For this review, take the finished solid that the model builds, in its own axes (mm). A direction names the side the tool comes from. Give positions to 0.01 mm unless a question says otherwise; leave off trailing zeros. Loops run counter-clockwise (first coordinate to the right, second up) from the corner with the lowest first, then second, coordinate; pieces in that order, holes last. Notation, with made-up numbers: (76, 10.25) -> (133, 10.25) arc R29 ccw to (133, 32.25) -> close; hole circle Ø1 at (21, 87). An arc over 180 degrees is marked (long way). Answer as CSV lines item,"result". Start each with the question number.
Item 1: Add section A-A on z = -142. State the section outline as (x, y) points.
Item 2: Clearance check with flat-ended pins moving along their axes: P1, Ø11.5, axis at y = 10, z = -51, coming from the +X side; P2, Ø4, axis at x = 6.5, z = -28, coming from the +Y side; P3, Ø2, axis at x = 13.5, z = -78.5, coming from the +Y side. State where each tip first meets the part, or that it passes through.
Item 3: The part is to be moulded in two halves that separate along X. For faces 1 (the face through (14, 23, 5)), 2 (the face through (-7.1, 22.18, 7.14)), 3 (the face through (2, 18, -180.976)), say which applies: +X half, -X half, draft (parallel to the pull), parting line (faces both ways), or undercut.
Item 4: Add section B-B on y = 7.5. State the section outline as (x, z) points.
Item 5: Add section C-C on x = 3. State the section outline as (y, z) points.
Item 6: Machinability: for faces 4 (the face through (0, 41, -92)), 5 (the face through (17.03, 18.25, -7.75)), 6 (the face through (19.976, 18, -2)), 7 (the face through (7.701, 18.252, -177.946)), which of the approach directions +Z, -Z, +X, -X, +Y, -Y give a long, thin tool a straight path to every point of the face, cutting with its end or side? Answer none if there is none.
Item 7: For L1, parallel to X at y = 11, z = -124.5; L2, parallel to Y at x = 0.5, z = -120.5; L3, parallel to Z at x = -3.75, y = 22, list the stretches that pass through material, from the lowest coordinate up. Write a range as from..to.
```python
from build123d import *

# Parameters (mm, degrees)
SKETCH_1_W                = 270
SKETCH_1_H                = 370
SKETCH_1_W_2              = 250
SKETCH_1_H_2              = 350
EXTRUDE_2_DEPTH           = 45
SKETCH_4_W                = 250
SKETCH_4_H                = 350
SKETCH_4_W_2              = 222
SKETCH_4_H_2              = 322
EXTRUDE_3_DEPTH           = 5
SKETCH_9_W                = 246
SKETCH_9_H                = 346
SKETCH_9_W_2              = 226
SKETCH_9_H_2              = 326
CUT_EXTRUDE_3_DEPTH       = 2.5
SKETCH_12_R               = 1.6
CUT_EXTRUDE_5_DEPTH       = 109.5
FILLET_1_R                = 5
SKETCH_13_W               = 250
SKETCH_13_H               = 350
SKETCH_13_W_2             = 222
SKETCH_13_H_2             = 322
EXTRUDE_4_DEPTH           = 33.5
CUT_EXTRUDE_START         = -126.5
SKETCH_14_R               = 1.6
CUT_EXTRUDE_9_DEPTH       = 126.5
SKETCH_15_R               = 1.6
CUT_EXTRUDE_10_DEPTH      = 50
CUT_EXTRUDE_11_DEPTH      = 2.5
CUT_EXTRUDE_12_DEPTH      = 188.55314569
CUT_EXTRUDE_12_DEPTH_BACK = 188.55314569


with BuildPart() as part:
    # 草图1 → 凸台-拉伸2 (new body)
    with BuildSketch(Plane(origin=(0, 0, 0), x_dir=(1, 0, 0), z_dir=(0, 1, 0))):
        with Locations((125, 175)):
            Rectangle(SKETCH_1_W, SKETCH_1_H)
        with Locations((125, 175)):
            Rectangle(SKETCH_1_W_2, SKETCH_1_H_2, mode=Mode.SUBTRACT)
    extrude(amount=EXTRUDE_2_DEPTH)

    # 草图4 → 凸台-拉伸3 (add)
    with BuildSketch(Plane(origin=(0, 38.5, 0), x_dir=(1, 0, 0), z_dir=(0, 1, 0))):
        with Locations((125, 175)):
            Rectangle(SKETCH_4_W, SKETCH_4_H)
        with Locations((125, 175)):
            Rectangle(SKETCH_4_W_2, SKETCH_4_H_2, mode=Mode.SUBTRACT)
    extrude(amount=-EXTRUDE_3_DEPTH)

    # 草图9 → 切除-拉伸3 (cut)
    with BuildSketch(Plane(origin=(0, 38.5, 0), x_dir=(1, 0, 0), z_dir=(0, 1, 0))):
        with Locations((125, 175)):
            Rectangle(SKETCH_9_W, SKETCH_9_H)
        with Locations((125, 175)):
            Rectangle(SKETCH_9_W_2, SKETCH_9_H_2, mode=Mode.SUBTRACT)
    extrude(amount=-CUT_EXTRUDE_3_DEPTH, mode=Mode.SUBTRACT)

    # 草图12 → 切除-拉伸5 (cut)
    with BuildSketch(Plane(origin=(0, 45, 0), x_dir=(1, 0, 0), z_dir=(0, 1, 0))):
        with Locations(Location((-3.535533906, -3.535533906, 0), (0, 0, 270))):
            Circle(SKETCH_12_R)
        with BuildLine():
            ThreePointArc((-4.666904756, 354.666904756), (-4.666904756, 352.404163056), (-2.404163056, 352.404163056))
            Line((-2.404163056, 352.404163056), (-4.666904756, 354.666904756))
        make_face()
        with BuildLine():
            Line((-4.666904756, 354.666904756), (-2.404163056, 352.404163056))
            ThreePointArc((-2.404163056, 352.404163056), (-2.057326654, 352.923240414), (-1.935533906, 353.535533906))
            ThreePointArc((-1.935533906, 353.535533906), (-2.923240414, 355.013741158), (-4.666904756, 354.666904756))
        make_face()
        with Locations(Location((253.535533906, 353.535533906, 0), (0, 0, 270))):
            Circle(SKETCH_12_R)
        with Locations(Location((253.535533906, -3.535533906, 0), (0, 0, 270))):
            Circle(SKETCH_12_R)
    extrude(amount=-CUT_EXTRUDE_5_DEPTH, mode=Mode.SUBTRACT)

    # 圆角1
    fillet_1_edges = [part.edges().sort_by_distance(p)[0] for p in [
        (-10, 22.5, 10),
        (-10, 22.5, -360),
        (260, 22.5, -360),
        (260, 22.5, 10),
    ]]
    fillet(fillet_1_edges, radius=FILLET_1_R)

    # 草图13 → 凸台-拉伸4 (add)
    with BuildSketch(Plane.XZ.offset(-33.5)):
        with Locations((125, -175)):
            Rectangle(SKETCH_13_W, SKETCH_13_H)
        with Locations((125, -175)):
            Rectangle(SKETCH_13_W_2, SKETCH_13_H_2, mode=Mode.SUBTRACT)
    extrude(amount=EXTRUDE_4_DEPTH)

    # 草图14 → 切除-拉伸9 (cut)
    # profile 1 of 8: a face of its own
    with BuildSketch(Plane.XZ.offset(CUT_EXTRUDE_START)):
        with BuildLine():
            Line((14, -336), (14, -175))
            Line((14, -175), (6, -175))
            Line((6, -175), (9.45, -180.975575286))
            Line((9.45, -180.975575286), (-5.45, -180.975575286))
            Line((-5.45, -180.975575286), (-2, -175))
            Line((-2, -175), (-10, -175))
            Line((-10, -175), (-10, -355))
            ThreePointArc((-10, -355), (-8.535533906, -358.535533906), (-5, -360))
            Line((-5, -360), (14, -360))
            Line((14, -360), (14, -352))
            Line((14, -352), (14, -344))
            Line((14, -344), (14, -336))
        make_face()
        with Locations((-3.535533906, -353.535533906)):
            Circle(SKETCH_14_R, mode=Mode.SUBTRACT)
    # profile 2 of 8: a face of its own
    with BuildSketch(Plane.XZ.offset(CUT_EXTRUDE_START)):
        Polygon((14, -6), (14, -14), (125, -14), (125, 10), (14, 10), (14, 2), (19.975575286, 5.45), (19.975575286, -9.45), align=None)
    # profile 3 of 8: a face of its own
    with BuildSketch(Plane.XZ.offset(CUT_EXTRUDE_START)):
        Polygon((125, 10), (125, -14), (236, -14), (236, -6), (230.024424714, -9.45), (230.024424714, 5.45), (236, 2), (236, 10), align=None)
    # profile 4 of 8: a face of its own
    with BuildSketch(Plane.XZ.offset(CUT_EXTRUDE_START)):
        with BuildLine():
            Line((236, -336), (14, -336))
            Line((14, -336), (14, -344))
            Line((14, -344), (19.975575286, -340.55))
            Line((19.975575286, -340.55), (19.975575286, -355.45))
            Line((19.975575286, -355.45), (14, -352))
            Line((14, -352), (14, -360))
            Line((14, -360), (255, -360))
            ThreePointArc((255, -360), (258.535533906, -358.535533906), (260, -355))
            Line((260, -355), (260, 5))
            ThreePointArc((260, 5), (258.535533906, 8.535533906), (255, 10))
            Line((255, 10), (236, 10))
            Line((236, 10), (236, 2))
            Line((236, 2), (236, -6))
            Line((236, -6), (236, -14))
            Line((236, -14), (236, -336))
        make_face()
        with Locations((253.535533906, -353.535533906)):
            Circle(SKETCH_14_R, mode=Mode.SUBTRACT)
        with Locations((253.535533906, 3.535533906)):
            Circle(SKETCH_14_R, mode=Mode.SUBTRACT)
    # profile 5 of 8: a face of its own
    with BuildSketch(Plane.XZ.offset(CUT_EXTRUDE_START)):
        Polygon((230.024424714, -9.45), (236, -6), (236, 2), (230.024424714, 5.45), align=None)
    # profile 6 of 8: a face of its own
    with BuildSketch(Plane.XZ.offset(CUT_EXTRUDE_START)):
        with Locations((253.535533906, -353.535533906)):
            Circle(SKETCH_14_R)
    # profile 7 of 8: a face of its own
    with BuildSketch(Plane.XZ.offset(CUT_EXTRUDE_START)):
        Polygon((19.975575286, -340.55), (14, -344), (14, -352), (19.975575286, -355.45), align=None)
    # profile 8 of 8: a face of its own
    with BuildSketch(Plane.XZ.offset(CUT_EXTRUDE_START)):
        with Locations((-3.535533906, -353.535533906)):
            Circle(SKETCH_14_R)
    extrude(amount=CUT_EXTRUDE_9_DEPTH, mode=Mode.SUBTRACT)

    # 草图15 → 切除-拉伸10 (cut)
    with BuildSketch(Plane(origin=(0, 45, 0), x_dir=(1, 0, 0), z_dir=(0, 1, 0))):
        with Locations(Location((-3.535533906, 76.464466094, 0), (0, 0, 270))):
            Circle(SKETCH_15_R)
    extrude(amount=-CUT_EXTRUDE_10_DEPTH, mode=Mode.SUBTRACT)

    # 草图16 → 切除-拉伸11 (cut)
    with BuildSketch(Plane(origin=(0, 38.5, 0), x_dir=(1, 0, 0), z_dir=(0, 1, 0))):
        Polygon((0, 0), (19.975575286, 0), (19.975575286, 2), (2, 2), (2, 180.975575286), (0, 180.975575286), align=None)
    extrude(amount=-CUT_EXTRUDE_11_DEPTH, mode=Mode.SUBTRACT)

    # 草图18 → 切除-拉伸12 (cut, two sides: drawn at the far end of the back side and taken through both)
    with BuildSketch(Plane(origin=(0, 45, 0), x_dir=(1, 0, 0), z_dir=(0, 1, 0)).offset(-CUT_EXTRUDE_12_DEPTH_BACK)):
        with BuildLine():
            Line((14, -10), (14, -8))
            Line((14, -8), (12, -8))
            Line((12, -8), (-5, -8))
            ThreePointArc((-5, -8), (-7.121320344, -7.121320344), (-8, -5))
            Line((-8, -5), (-8, 173))
            Line((-8, 173), (-8, 175))
            Line((-8, 175), (-10, 175))
            Line((-10, 175), (-10, -5))
            ThreePointArc((-10, -5), (-8.535533906, -8.535533906), (-5, -10))
            Line((-5, -10), (14, -10))
        make_face()
    extrude(amount=CUT_EXTRUDE_12_DEPTH + CUT_EXTRUDE_12_DEPTH_BACK, mode=Mode.SUBTRACT)


solid = part.part
```
Computed values:
1,outline,"(-8, 0) -> (14, 0) -> (14, 38.5) -> (12, 38.5) -> (12, 36) -> (0, 36) -> (0, 45) -> (-8, 45) -> close"
2,P1,"x = 14"
2,P2,"y = 36"
2,P3,"y = 38.5"
3,face 1,"undercut"
3,face 2,"-X half"
3,face 3,"draft"
4,outline,"(-8, -175) -> (-2, -175) -> (-5.45, -180.98) -> (9.45, -180.98) -> (6, -175) -> (14, -175) -> (14, -6) -> (19.98, -9.45) -> (19.98, 5.45) -> (14, 2) -> (14, 8) -> (-5, 8) arc R3 ccw to (-8, 5) -> close; hole circle Ø3.2 at (-3.54, -76.46); hole circle Ø3.2 at (-3.54, 3.54)"
5,outline,"(0, -180.98) -> (36, -180.98) -> (36, 0) -> (45, 0) -> (45, 8) -> (0, 8) -> close"
6,face 4,"-Z, +Y"
6,face 5,"-Z, +Y, -Y"
6,face 6,"+Z, -Z, +X, +Y, -Y"
6,face 7,"+X, +Y, -Y"
7,L1,"-8..14"
7,L2,"0..36"
7,L3,"-180.98..-178.03, -175..-78.05, -74.88..1.95, 5.12..8"
